from build123d import *

# Parameters (mm, degrees)
SKETCH_W        = 126
SKETCH_H        = 140
PAD_DEPTH       = 50
SKETCH002_W     = 120
SKETCH002_H     = 134
POCKET_DEPTH    = 47
SKETCH001_W     = 10
SKETCH001_H     = 14
SKETCH001_W_2   = 3.4
SKETCH001_H_2   = 7.25
PAD001_DEPTH    = 61
SKETCH003_R     = 2.3
POCKET001_DEPTH = 123.001
SKETCH004_R     = 4.5
PAD002_DEPTH    = 5
SKETCH005_R     = 2.2
POCKET002_DEPTH = 8.001
CHAMFER_SIZE    = 2
CHAMFER001_SIZE = 0.35
CHAMFER002_SIZE = 1
CHAMFER003_SIZE = 0.75
CHAMFER004_SIZE = 1
CHAMFER005_SIZE = 2


with BuildPart() as part:
    # Sketch → Pad (new body)
    with BuildSketch(Plane.XY):
        Rectangle(SKETCH_W, SKETCH_H)
    extrude(amount=PAD_DEPTH)

    # Sketch002 → Pocket (cut)
    with BuildSketch(Plane.XY.offset(50)):
        Rectangle(SKETCH002_W, SKETCH002_H)
    extrude(amount=-POCKET_DEPTH, mode=Mode.SUBTRACT)

    # Sketch001 → Pad001 (new body)
    with BuildSketch(Plane.XY.offset(3)):
        with Locations((-55, 45)):
            Rectangle(SKETCH001_W, SKETCH001_H)
        with Locations((-55, 45)):
            Rectangle(SKETCH001_W_2, SKETCH001_H_2, mode=Mode.SUBTRACT)
        with Locations((55, 45)):
            Rectangle(SKETCH001_W, SKETCH001_H)
        with Locations((55, 45)):
            Rectangle(SKETCH001_W_2, SKETCH001_H_2, mode=Mode.SUBTRACT)
        with Locations((-55, -45)):
            Rectangle(SKETCH001_W, SKETCH001_H)
        with Locations((-55, -45)):
            Rectangle(SKETCH001_W_2, SKETCH001_H_2, mode=Mode.SUBTRACT)
        with Locations((55, -45)):
            Rectangle(SKETCH001_W, SKETCH001_H)
        with Locations((55, -45)):
            Rectangle(SKETCH001_W_2, SKETCH001_H_2, mode=Mode.SUBTRACT)
    extrude(amount=PAD001_DEPTH)

    # Sketch003 → Pocket001 (cut, through all)
    with BuildSketch(Plane.YZ.offset(60)):
        with Locations((-45, 58)):
            Circle(SKETCH003_R)
        with Locations((45, 58)):
            Circle(SKETCH003_R)
    extrude(amount=-POCKET001_DEPTH, mode=Mode.SUBTRACT)

    # Sketch004 → Pad002 (new body)
    with BuildSketch(Plane.XY.offset(3)):
        with Locations((-38.1655, 50.887)):
            Circle(SKETCH004_R)
        with Locations((38.1655, 50.887)):
            Circle(SKETCH004_R)
        with Locations((-38.1655, -50.887)):
            Circle(SKETCH004_R)
        with Locations((38.1655, -50.887)):
            Circle(SKETCH004_R)
    extrude(amount=PAD002_DEPTH)

    # Sketch005 → Pocket002 (cut, through all)
    with BuildSketch(Plane.XY.offset(8)):
        with Locations((-38.1655, 50.887)):
            Circle(SKETCH005_R)
        with Locations((38.1655, 50.887)):
            Circle(SKETCH005_R)
        with Locations((-38.1655, -50.887)):
            Circle(SKETCH005_R)
        with Locations((38.1655, -50.887)):
            Circle(SKETCH005_R)
    extrude(amount=-POCKET002_DEPTH, mode=Mode.SUBTRACT)

    # Chamfer
    chamfer_edges = [part.edges().sort_by_distance(p)[0] for p in [
        (63, 0, 0),
        (0, 70, 0),
        (0, -70, 0),
        (-63, 0, 0),
    ]]
    chamfer(chamfer_edges, length=CHAMFER_SIZE)

    # Chamfer001
    chamfer001_edges = [part.edges().sort_by_distance(p)[0] for p in [
        (-40.3655, -50.887, 0),
        (35.9655, -50.887, 0),
        (35.9655, 50.887, 0),
        (-40.3655, 50.887, 0),
    ]]
    chamfer(chamfer001_edges, length=CHAMFER001_SIZE)

    # Chamfer002
    chamfer002_edges = [part.edges().sort_by_distance(p)[0] for p in [
        (-55, 52, 64),
        (-50, 45, 64),
        (-55, 38, 64),
        (-60, 45, 64),
        (-55, 48.625, 64),
        (-53.3, 45, 64),
        (-55, 41.375, 64),
        (-56.7, 45, 64),
        (-55, -38, 64),
        (-50, -45, 64),
        (-55, -52, 64),
        (-60, -45, 64),
        (-55, -41.375, 64),
        (-53.3, -45, 64),
        (-55, -48.625, 64),
        (-56.7, -45, 64),
        (55, 52, 64),
        (60, 45, 64),
        (55, 38, 64),
        (50, 45, 64),
        (55, 48.625, 64),
        (56.7, 45, 64),
        (55, 41.375, 64),
        (53.3, 45, 64),
        (55, -38, 64),
        (60, -45, 64),
        (55, -52, 64),
        (50, -45, 64),
        (55, -41.375, 64),
        (56.7, -45, 64),
        (55, -48.625, 64),
        (53.3, -45, 64),
    ]]
    chamfer(chamfer002_edges, length=CHAMFER002_SIZE)

    # Chamfer003
    chamfer003_edges = [part.edges().sort_by_distance(p)[0] for p in [
        (-60, 42.7, 58),
        (-60, -47.3, 58),
        (50, -47.3, 58),
        (50, 42.7, 58),
        (-50, 42.7, 58),
        (60, 42.7, 58),
        (60, -47.3, 58),
        (-50, -47.3, 58),
    ]]
    chamfer(chamfer003_edges, length=CHAMFER003_SIZE)

    # Chamfer004
    chamfer004_edges = [part.edges().sort_by_distance(p)[0] for p in [
        (-63, 70, 26),
        (63, 70, 26),
        (63, -70, 26),
        (-63, -70, 26),
    ]]
    chamfer(chamfer004_edges, length=CHAMFER004_SIZE)

    # Chamfer005
    chamfer005_edges = [part.edges().sort_by_distance(p)[0] for p in [
        (-60, -67, 26.5),
        (0, -67, 3),
        (-60, 0, 3),
        (0, 67, 3),
        (60, 0, 3),
        (-60, 67, 26.5),
        (60, 67, 26.5),
        (60, 59.5, 3),
        (-60, 59.5, 3),
        (60, -59.5, 3),
        (-60, -59.5, 3),
    ]]
    chamfer(chamfer005_edges, length=CHAMFER005_SIZE)


solid = part.part
Work out the finished part from the listing and answer in its coordinate system (mm). A direction names the side the tool comes from. Give positions to 0.01 mm unless a question says otherwise; leave off trailing zeros. Write each loop counter-clockwise with the first axis right and the second up, starting at its lowest first coordinate (ties: lowest second). Pieces come first, ordered by that corner, then holes. Notation, with made-up numbers: (74, 45.25) - (91, 45.25) arc R10 cw to (91, 55.25) - close; hole circle Ø10 at (0.25, 58). An arc over 180 degrees is marked (long way). One line per item, written item: value. Start each with the question number.
1. Consider probe 1 along X at (y, z) = (-46, 38.5); probe 2 along X at (y, z) = (22, 10); probe 3 along Y at (x, z) = (33, 32). Determine where each line is inside the solid, lowest interval first.
2. For faces 5 (the flat face through (0, -67, 28)), 6 (the flat face through (-1, 1, 0)), 7 (the flat face through (60, 43, 55)), determine the directions among +Z, -Z, +X, -X, +Y, -Y from which every point of the face is accessible in a straight line to the end or side of a thin tool.
3. Find section A-A (x = -20). Write down the section's boundary in (y, z), then the cut area to 3 significant figures.
4. For a pull along Z with two mould halves and no side action, classify faces 1 (the cylindrical face through (-52.007, -45.499, 55.755)), 2 (the flat face through (-58, 45, 64)), 3 (the cylindrical face through (52.043, -45.499, 55.755)), 4 (the flat face through (-1, -70, 26)) as +Z half, -Z half, draft (parallel to the pull), parting line (faces both ways), or undercut.
5. Find section B-B (y = -26.5). Write down the section's boundary in (x, z).
6. Given pin 1 (5 mm diameter, centred on x = -38.17, y = 50.89, fed in from -Z); pin 2 (3.5 mm diameter, centred on x = -54.5, y = -44.5, fed in from +Z); pin 3 (7 mm diameter, centred on x = -40, y = 50, fed in from +Z), each flat-ended and moving along its own axis, determine where each tip first touches the part or whether it passes through.
7. Find section C-C (z = 58). State how many separate pieces and enclosed holes the cut face has, then the cut area to 3 significant figures.
Geometry results:
1. probe 1: -63 to -56.7, -53.3 to -50, 50 to 53.3, 56.7 to 63
1. probe 2: -63 to -60, 60 to 63
1. probe 3: -70 to -67, 67 to 70
2. face 5: +Z
2. face 6: -Z, +X, -X, +Y, -Y
2. face 7: +Z, +X, +Y, -Y
3. outline: (-70, 2) - (-68, 0) - (68, 0) - (70, 2) - (70, 50) - (67, 50) - (67, 5) - (65, 3) - (-65, 3) - (-67, 5) - (-67, 50) - (-70, 50) - close
3. area: 702 mm2
4. face 1: undercut
4. face 2: +Z half
4. face 3: undercut
4. face 4: draft
5. outline: (-63, 2) - (-61, 0) - (61, 0) - (63, 2) - (63, 50) - (60, 50) - (60, 5) - (58, 3) - (-58, 3) - (-60, 5) - (-60, 50) - (-63, 50) - close
6. pin 1: z = 0.04
6. pin 2: z = 63.55
6. pin 3: z = 8
7. separate pieces: 8
7. enclosed holes: 0
7. area: 335 mm2
